Answer from the drawing. Dimensions are ordinates in mm from the lowest x, y and z of the part. A direction names the side the tool comes from. Give positions to 0.01 mm unless a question says otherwise; leave off trailing zeros. Loops run counter-clockwise (first coordinate to the right, second up) from the corner with the lowest first, then second, coordinate; pieces in that order, holes last. Notation, with made-up numbers: (76.5, 85) -> (97.5, 85) arc R19 cw to (97.5, 104) -> close; hole circle Ø7 at (52, 13). An arc over 180 degrees is marked (long way). Return JSON: item names as keys, results as strings. Group by question number.
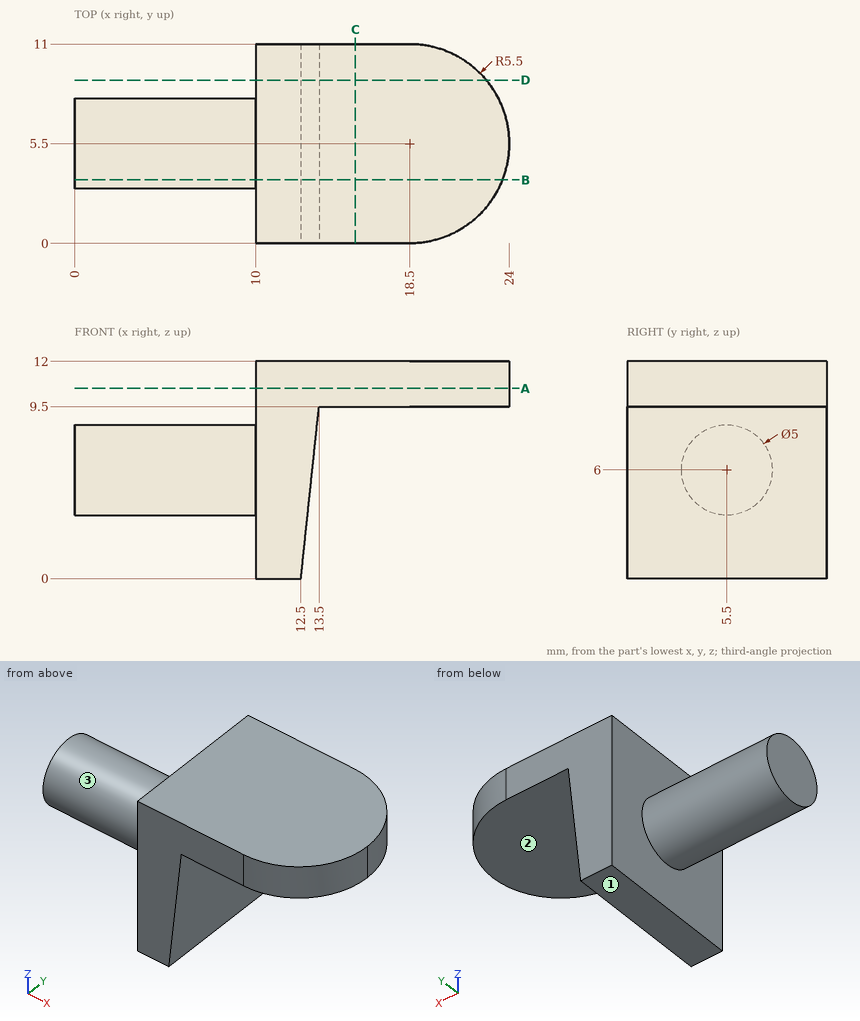
1. Section D-D on y = 9 is taken. Determine the outline of the cut face in (x, z).
2. Section B-B on y = 3.5 is taken. Determine the outline of the cut face in (x, z).
3. Section C-C on x = 15.5 is taken. Determine the outline of the cut face in (y, z), then the cut area to 3 significant figures.
4. Which of the six approach directions +Z, -Z, +X, -X, +Y, -Y give full straight-line access (tool end or side, diameter ignored) to the marked faces 1, 2 and 3?
5. Straight lines are drawn through the part: line 1 (Z direction, x = 21, y = 4.25); line 2 (X direction, y = 1, z = 5.75); line 3 (Z direction, x = 3, y = 7.75). For each, find the intervals that lie inside material, in ascending order. Write a range as from..to.
6. Section A-A on z = 10.5 is taken. Determine the outline of the cut face in (x, y), then the cut area to 3 significant figures.
7. Flat-ended cylindrical pins translate along their axes: pin 1 Ø6 at (y, z) = (2, 8.5) entering from +X; pin 2 Ø6 at (y, z) = (6.5, 4) entering from +X; pin 3 Ø5 at (x, y) = (17, 4) entering from -Z; pin 4 Ø1.5 at (x, z) = (8, 11) entering from -Y. Find the tip coordinate at first contact, or state that the pin passes through.
Completed:
{
 "1": {"outline": "(10, 0) -> (12.5, 0) -> (13.5, 9.5) -> (22.74, 9.5) -> (22.74, 12) -> (10, 12) -> close"},
 "2": {"outline": "(0, 4.5) -> (10, 4.5) -> (10, 0) -> (12.5, 0) -> (13.5, 9.5) -> (23.62, 9.5) -> (23.62, 12) -> (10, 12) -> (10, 7.5) -> (0, 7.5) -> close"},
 "3": {"outline": "(0, 9.5) -> (11, 9.5) -> (11, 12) -> (0, 12) -> close", "area": "27.5 mm²"},
 "4": {"face 1": "-Z, +X, -X, +Y, -Y", "face 2": "-Z, +X, +Y, -Y", "face 3": "-X"},
 "5": {"line 1": "z = 9.5..12", "line 2": "x = 10..13.11", "line 3": "z = 4.91..7.09"},
 "6": {"outline": "(10, 0) -> (18.5, 0) arc R5.5 ccw to (18.5, 11) -> (10, 11) -> close", "area": "141 mm²"},
 "7": {"pin 1": "stops at x = 23.96", "pin 2": "stops at x = 13.24", "pin 3": "stops at z = 9.5", "pin 4": "passes through"}
}
